Verification items for the finished model (mm, model axes). Face numbers are marked on the shaded views. A direction names the side the tool comes from. Coordinates: 2 decimals unless noted, no trailing zeros. Loops run counter-clockwise (first coordinate to the right, second up) from the corner with the lowest first, then second, coordinate; pieces in that order, holes last. Notation, with made-up numbers: (-11.75, 85) -> (-7.75, 85) arc R26 ccw to (-7.75, 123) -> close; hole circle Ø8 at (-9.75, 79). An arc over 180 degrees is marked (long way). Answer as a JSON object with one key per item and string values. Group by question number.
Q1. Cross-section at B-B on z = 2.75. Record the boundary of the cut face in (x, y) (3 decimals), and give its area (3 significant figures).
Q2. Set-up check for the marked faces 1, 2 and 3: record each of +Z, -Z, +X, -X, +Y, -Y from which the full face is reachable in a straight line by a thin tool's end or side.
Q3. Cross-section at A-A on x = 3.75. Record the boundary of the cut face in (y, z).
Q4. Cross-section at C-C on y = -14. Record the boundary of the cut face in (x, z).
Q5. Gauge pin test, flat ends, axial feed: pin 1 Ø1.2 at (y, z) = (-14, 5.33) entering from +X; pin 2 Ø3 at (x, y) = (1, 1.5) entering from +Z; pin 3 Ø1.5 at (x, z) = (-1.5, 0.5) entering from -Y; pin 4 Ø1.6 at (x, y) = (0, -7) entering from -Z. Record the tip position at first contact, or that the pin passes through.
Q6. Scan lines: L1, parallel to X at y = -11, z = 1; L2, parallel to Y at x = -1.25, z = -1.5; L3, parallel to Y at x = 3.5, z = 7.25 (3 decimals). Record each from-to range of solid material in increasing order.
Q7. Cross-section at D-D on z = 0. Record the boundary of the cut face in (x, y), and give its area (4 significant figures).
Q8. Release check for a two-part mould opening along Y. For the marked faces 4, 5, 6 and 7 record: released by +Y, released by -Y, zero draft, split by the parting line, or undercut.
```python
from build123d import *

# Parameters (mm, degrees)
SKETCH4_W           = 10
SKETCH4_H           = 15
BOSS_EXTRUDE3_DEPTH = 2.5
SKETCH5_R           = 2.5
BOSS_EXTRUDE4_DEPTH = 6
SKETCH6_W           = 10
SKETCH6_H           = 5
BOSS_EXTRUDE5_DEPTH = 2
BOSS_EXTRUDE6_DEPTH = 2.5
BOSS_EXTRUDE7_DEPTH = 2.5
SKETCH9_R           = 0.75
CUT_EXTRUDE1_DEPTH  = 21.97683908


with BuildPart() as part:
    # Sketch4 → Boss-Extrude3 (new body)
    with BuildSketch(Plane(origin=(0, 0, 0), x_dir=(1, 0, 0), z_dir=(0, 1, 0))):
        Rectangle(SKETCH4_W, SKETCH4_H)
    extrude(amount=BOSS_EXTRUDE3_DEPTH)

    # Sketch5 → Boss-Extrude4 (add)
    with BuildSketch(Plane.XZ):
        with Locations(Location((0, 0, 0), (0, 0, 270))):
            Circle(SKETCH5_R)
    extrude(amount=BOSS_EXTRUDE4_DEPTH)

    # Sketch6 → Boss-Extrude5 (add)
    with BuildSketch(Plane.XZ.offset(6)):
        Rectangle(SKETCH6_W, SKETCH6_H)
    extrude(amount=BOSS_EXTRUDE5_DEPTH)

    # Sketch7 → Boss-Extrude6 (add)
    with BuildSketch(Plane.ZY.offset(5)):
        Polygon((-2.5, -6), (2.5, -6), (9.166666667, -16), (4.166666667, -16), align=None)
    extrude(amount=-BOSS_EXTRUDE6_DEPTH)

    # Sketch8 → Boss-Extrude7 (add)
    with BuildSketch(Plane(origin=(5, 0, 0), x_dir=(0, 0, -1), z_dir=(1, 0, 0))):
        Polygon((2.5, -6), (-2.5, -6), (-9.166666667, -16), (-4.166666667, -16), align=None)
    extrude(amount=-BOSS_EXTRUDE7_DEPTH)

    # Sketch9 → Cut-Extrude1 (cut, through all)
    with BuildSketch(Plane.ZY.offset(5)):
        with Locations((5.333333333, -14)):
            Circle(SKETCH9_R)
    extrude(amount=-CUT_EXTRUDE1_DEPTH, mode=Mode.SUBTRACT)


solid = part.part
```
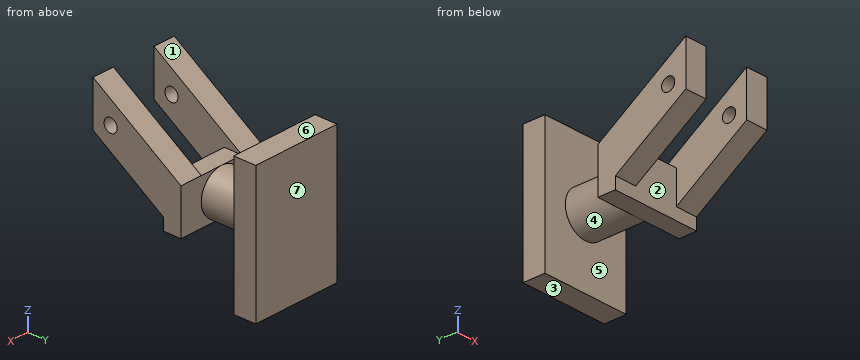
Computed values:
{
 "1": {"outline": "(-5, -13.875) -> (-2.5, -13.875) -> (-2.5, -6.375) -> (-5, -6.375) -> close; (-5, 0) -> (5, 0) -> (5, 2.5) -> (-5, 2.5) -> close; (2.5, -13.875) -> (5, -13.875) -> (5, -6.375) -> (2.5, -6.375) -> close", "area": "62.5 mm²"},
 "2": {"face 1": "+Z, +X, -X", "face 2": "-Z, -Y", "face 3": "-Z, +X, -X, +Y, -Y"},
 "3": {"outline": "(-16, 4.17) -> (-8, -1.17) -> (-8, -2.5) -> (-6, -2.5) -> (-6, 2.5) -> (-16, 9.17) -> close; (0, -7.5) -> (2.5, -7.5) -> (2.5, 7.5) -> (0, 7.5) -> close; hole circle Ø1.5 at (-14, 5.33)"},
 "4": {"outline": "(-5, 2.83) -> (-2.5, 2.83) -> (-2.5, 4.58) -> (-5, 4.58) -> close; (-5, 6.08) -> (-2.5, 6.08) -> (-2.5, 7.83) -> (-5, 7.83) -> close; (2.5, 2.83) -> (5, 2.83) -> (5, 4.58) -> (2.5, 4.58) -> close; (2.5, 6.08) -> (5, 6.08) -> (5, 7.83) -> (2.5, 7.83) -> close"},
 "5": {"pin 1": "passes through", "pin 2": "stops at z = 7.5", "pin 3": "stops at y = -8", "pin 4": "stops at z = -2.5"},
 "6": {"L1": "x = -5 to -2.5, 2.5 to 5", "L2": "y = -8 to 2.5", "L3": "y = -16 to -13.125, 0 to 2.5"},
 "7": {"outline": "(-5, -9.75) -> (-2.5, -9.75) -> (-2.5, -8) -> (2.5, -8) -> (2.5, -9.75) -> (5, -9.75) -> (5, -6) -> (2.5, -6) -> (2.5, 0) -> (5, 0) -> (5, 2.5) -> (-5, 2.5) -> (-5, 0) -> (-2.5, 0) -> (-2.5, -6) -> (-5, -6) -> close", "area": "83.75 mm²"},
 "8": {"face 4": "undercut", "face 5": "undercut", "face 6": "zero draft", "face 7": "released by +Y"}
}
